from build123d import *

# Parameters (mm, degrees)
F0_W     = 10
F0_H     = 10
F0_W_2   = 0.086959
F1_DEPTH = 10


with BuildPart() as f1:
    # F0 (on Top) → F1 (new body)
    with BuildSketch(Plane.XY):
        with Locations((-140, -60)):
            Rectangle(F0_W, F0_H)
        with Locations((-150, 50)):
            Rectangle(F0_W, F0_H)
        Polygon((-155, 25), (-145.130813, 25), (-145, 25), (-145, 35), (-155, 35), align=None)
        Polygon((-155, 5), (-145, 5), (-145, 15), (-145.130813, 15), (-155, 15), align=None)
        with Locations((-150, -10)):
            Rectangle(F0_W, F0_H)
        with Locations((-150, -30)):
            Rectangle(F0_W, F0_H)
        Polygon((-155, -55), (-145.086959, -55), (-145, -55), (-145, -45), (-155, -45), align=None)
        with Locations((150, -50)):
            Rectangle(F0_W, F0_H)
        with Locations((-140, 60)):
            Rectangle(F0_W, F0_H)
        with Locations((-120, 60)):
            Rectangle(F0_W, F0_H)
        with Locations((-100, 60)):
            Rectangle(F0_W, F0_H)
        with Locations((-80, 60)):
            Rectangle(F0_W, F0_H)
        with Locations((-60, 60)):
            Rectangle(F0_W, F0_H)
        with Locations((-40, 60)):
            Rectangle(F0_W, F0_H)
        with Locations((-20, 60)):
            Rectangle(F0_W, F0_H)
        Polygon((-5, 65), (-5, 55), (-5, 54.502327), (5, 54.502327), (5, 55), (5, 65), align=None)
        with Locations((20, 60)):
            Rectangle(F0_W, F0_H)
        with Locations((40, 60)):
            Rectangle(F0_W, F0_H)
        with Locations((60, 60)):
            Rectangle(F0_W, F0_H)
        Polygon((75, 65), (75, 55), (85, 55), (85, 55.006977), (85, 65), align=None)
        Polygon((95, 65), (95, 55.006977), (95, 55), (105, 55), (105, 65), align=None)
        with Locations((120, 60)):
            Rectangle(F0_W, F0_H)
        with Locations((140, 60)):
            Rectangle(F0_W, F0_H)
        with Locations((-120, -60)):
            Rectangle(F0_W, F0_H)
        with Locations((-100, -60)):
            Rectangle(F0_W, F0_H)
        with Locations((-80, -60)):
            Rectangle(F0_W, F0_H)
        with Locations((-60, -60)):
            Rectangle(F0_W, F0_H)
        with Locations((-40, -60)):
            Rectangle(F0_W, F0_H)
        with Locations((-20, -60)):
            Rectangle(F0_W, F0_H)
        with Locations((0, -60)):
            Rectangle(F0_W, F0_H)
        with Locations((20, -60)):
            Rectangle(F0_W, F0_H)
        with Locations((40, -60)):
            Rectangle(F0_W, F0_H)
        with Locations((60, -60)):
            Rectangle(F0_W, F0_H)
        with Locations((80, -60)):
            Rectangle(F0_W, F0_H)
        with Locations((100, -60)):
            Rectangle(F0_W, F0_H)
        with Locations((120, -60)):
            Rectangle(F0_W, F0_H)
        with Locations((140, -60)):
            Rectangle(F0_W, F0_H)
        with Locations((150, 50)):
            Rectangle(F0_W, F0_H)
        with Locations((150, 30)):
            Rectangle(F0_W, F0_H)
        with Locations((150, 10)):
            Rectangle(F0_W, F0_H)
        with Locations((150, -10)):
            Rectangle(F0_W, F0_H)
        with Locations((150, -30)):
            Rectangle(F0_W, F0_H)
        Polygon((-145, -45), (-145, -55), (-135, -55), (-125, -55), (-115, -55), (-105, -55), (-95, -55), (-85, -55), (-75, -55), (-65, -55), (-55, -55), (-45, -55), (-35, -55), (-25, -55), (-15, -55), (-5, -55), (5, -55), (15, -55), (25, -55), (35, -55), (45, -55), (55, -55), (65, -55), (75, -55), (85, -55), (95, -55), (105, -55), (115, -55), (125, -55), (135, -55), (145, -55), (145, -45), (145, -35), (145, -25), (145, -15), (145, -5), (145, 5), (145, 15), (145, 25), (145, 35), (145, 45), (145, 55), (135, 55), (125, 55), (115, 55), (105, 55), (95, 55), (95, 55.006977), (85, 55.006977), (85, 55), (75, 55), (65, 55), (55, 55), (45, 55), (35, 55), (25, 55), (15, 55), (5, 55), (5, 54.502327), (-5, 54.502327), (-5, 55), (-15, 55), (-25, 55), (-35, 55), (-45, 55), (-55, 55), (-65, 55), (-75, 55), (-85, 55), (-95, 55), (-105, 55), (-115, 55), (-125, 55), (-135, 55), (-145, 55), (-145, 45), (-145, 35), (-145, 25), (-145.130813, 25), (-145.130813, 15), (-145, 15), (-145, 5), (-145, -5), (-145, -15), (-145, -25), (-145, -35), align=None)
        with Locations((-145.043479, -60)):
            Rectangle(F0_W_2, F0_H)
    extrude(amount=F1_DEPTH)


solid = f1.part
Here's how the part is built. I have some questions about the finished solid (model axes, mm). A direction names the side the tool comes from. Coordinates: 2 decimals unless noted, no trailing zeros. Write each loop counter-clockwise with the first axis right and the second up, starting at its lowest first coordinate (ties: lowest second). Pieces come first, ordered by that corner, then holes.
Item 1: If we mould it in two halves opening along Y, with no side actions, what happens to faces 4 (the flat face through (-70, -55, 5)), 5 (the flat face through (105, -60, 5)), 6 (the flat face through (-150, -35, 5))? For each: +Y half, -Y half, draft (parallel to the pull), parting line (faces both ways), or undercut.
Item 2: Will these pins go through, and if not, where does the flat tip stop? pin 1 (3 mm diameter, centred on y = 59, z = 3.5, fed in from -X); pin 2 (6 mm diameter, centred on y = 42.5, z = 2, fed in from -X); pin 3 (5 mm diameter, centred on y = -60, z = 2.5, fed in from +X); pin 4 (3 mm diameter, centred on y = -59, z = 3.5, fed in from -X).
Item 3: If I drill on line 1 (Y direction, x = -46.5, z = 4.5); line 2 (X direction, y = 36, z = 5.25), over which ranges is the centre line in solid material (lowest first)?
Item 4: I want a section at B-B on y = 21.5. Write out the boundary of the cut face in (x, z).
Item 5: On a 3-axis mill with a long thin cutter (end or side, diameter ignored), from which of +Z, -Z, +X, -X, +Y, -Y can I reach the whole of each face in a straight line? I mean faces 1 (the flat face through (-150, 5, 5)), 2 (the flat face through (-110, -55, 5)), 3 (the flat face through (75, 60, 5)). Say none if no direction works.
Item 6: I want a section at A-A on x = 68. Write out the boundary of the cut face in (y, z), and give its area (3 significant figures).
Findings below:
1. face 4: -Y half
1. face 5: draft
1. face 6: undercut
2. pin 1: stops at x = -145
2. pin 2: stops at x = -155
2. pin 3: stops at x = 145
2. pin 4: stops at x = -145.09
3. line 1: y = -55 to 55
3. line 2: x = -145 to 145
4. outline: (-145.13, 0) - (145, 0) - (145, 10) - (-145.13, 10) - close
5. face 1: +Z, -Z, -X
5. face 2: +Z, -Z, -Y
5. face 3: +Z, -Z, +Y
6. outline: (-55, 0) - (55, 0) - (55, 10) - (-55, 10) - close
6. area: 1,100 mm2
